Job drawing, mm, ordinate dimensions from the low corner. One solid piece. A direction names the side the tool comes from. Round coordinates to 2 decimals unless told otherwise and drop trailing zeros. Order: outer loops, then holes, each group sorted by start corner. A loop starts at its lowest first (then second) coordinate and runs counter-clockwise, first axis right, second up. Notation, with made-up numbers: (44, 76.25) -> (103, 76.25) arc R20 cw to (103, 101.25) -> close; hole circle Ø9 at (82.25, 51). An arc over 180 degrees is marked (long way). Use CSV: the item, a comma, the result in double quotes.
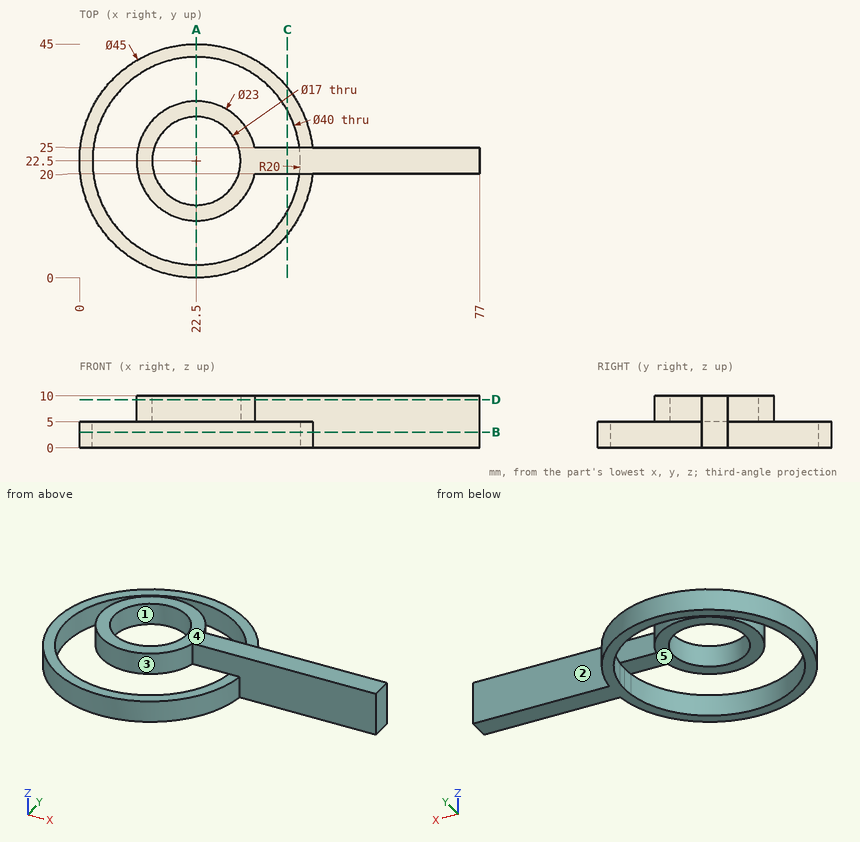
(1) Which spindle directions (+Z, -Z, +X, -X, +Y, -Y) get a long thin tool onto all of the face, cutting with end or side? Do the marked faces 4 and 5. Say none if no direction does.
Reply:
face 4,"+Z, +X, -X, +Y, -Y"
face 5,"-Z"
(2) Cut at A-A, the plane x = 22.5. Give the cut face in (y, z), then the cut area to 3 significant figures.
Reply:
outline,"(0, 0) -> (2.5, 0) -> (2.5, 5) -> (0, 5) -> close; (11, 5) -> (14, 5) -> (14, 10) -> (11, 10) -> close; (31, 5) -> (34, 5) -> (34, 10) -> (31, 10) -> close; (42.5, 0) -> (45, 0) -> (45, 5) -> (42.5, 5) -> close"
area,"55.0 mm2"
(3) Probe probe 1 along Y at (x, z) = (22.5, 2.2); probe 2 along Y at (x, z) = (22.5, 6.8); probe 3 along Y at (x, z) = (55, 6). List the from-to ranges inside material, lowest first. Write a range as [from, to].
Reply:
probe 1,"[0, 2.5], [42.5, 45]"
probe 2,"[11, 14], [31, 34]"
probe 3,"[20, 25]"
(4) Cut at D-D, the plane z = 9.25. Give the cut face in (x, y) (3 decimals), then the cut area to 3 significant figures.
Reply:
outline,"(33.725, 20) -> (77, 20) -> (77, 25) -> (33.725, 25) arc R11.5 ccw (long way) to start; hole circle Ø17 at (22.5, 22.5)"
area,"404 mm2"
(5) Drop flat-ended pins along their axis: P1, Ø3, axis at x = 52, z = 5.5, coming from the +Y side; P2, Ø18.5, axis at x = 22, y = 21.5, coming from the -Z side; P3, Ø6, axis at y = 23.5, z = 1, coming from the -X side; P4, Ø5, axis at x = 13, y = 37.5, coming from the -Z side. Give the stop position or say it passes through.
Reply:
P1,"y = 25"
P2,"z = 5"
P3,"x = 0"
P4,"z = 0"
(6) Cut at C-C, the plane x = 40. Give the cut face in (y, z), then the cut area to 3 significant figures.
Reply:
outline,"(8.36, 0) -> (12.82, 0) -> (12.82, 5) -> (8.36, 5) -> close; (20, 5) -> (25, 5) -> (25, 10) -> (20, 10) -> close; (32.18, 0) -> (36.64, 0) -> (36.64, 5) -> (32.18, 5) -> close"
area,"69.6 mm2"
(7) Pull direction Y, two halves, no side cores. Call the marked faces 1, 2 and 3: released by +Y, released by -Y, zero draft, split by the parting line, or undercut.
Reply:
face 1,"undercut"
face 2,"released by +Y"
face 3,"split by the parting line"
(8) Cut at B-B, the plane z = 3. Give the cut face in (x, y), then the cut area to 3 significant figures.
Reply:
outline,"(44.86, 20) -> (77, 20) -> (77, 25) -> (44.86, 25) arc R22.5 ccw (long way) to start; hole (42.34, 20) arc R20 ccw to (42.5, 22.5) arc R20 ccw to (42.34, 25) arc R20 ccw (long way) to start"
area,"494 mm2"
